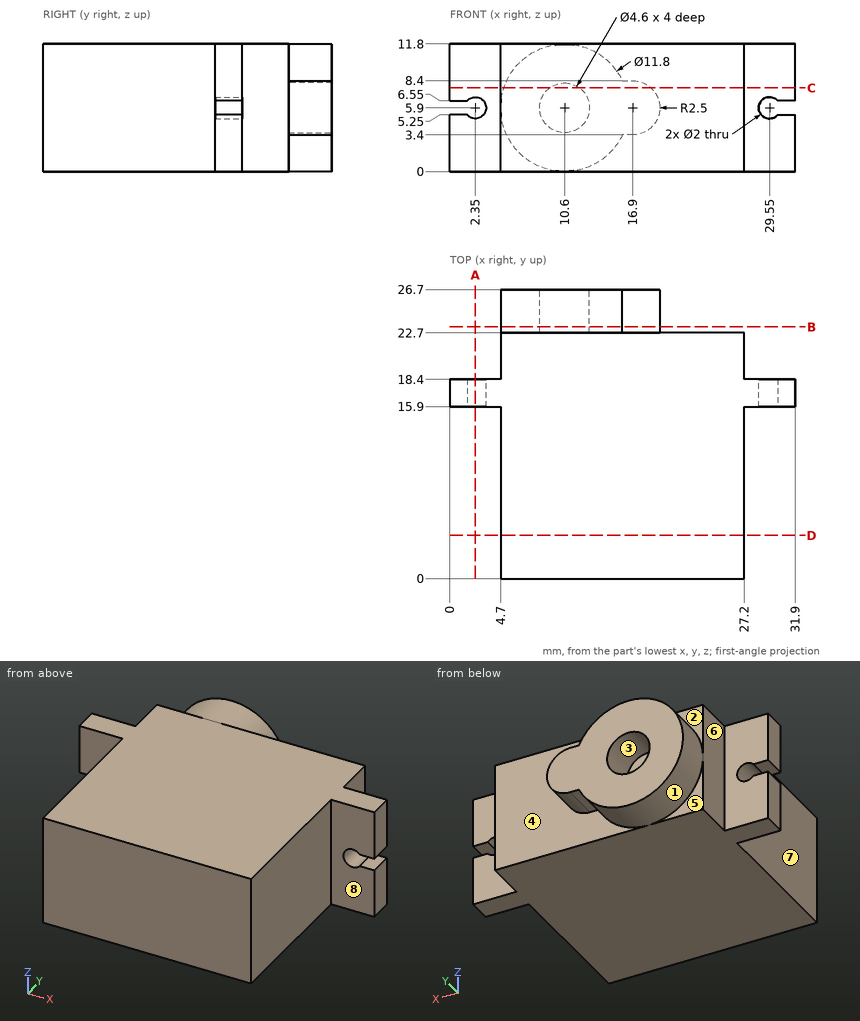
Design review of the part shown in the three views and the two pictorial views. Dimensions are in mm from the part's minimum x, y and z. A direction names the side the tool comes from. Round coordinates to 2 decimals unless told otherwise and drop trailing zeros. Write each loop counter-clockwise with the first axis right and the second up, starting at its lowest first coordinate (ties: lowest second). Pieces come first, ordered by that corner, then holes.
1) Take a section at C-C on z = 7.75. Give the boundary of the cut face in (x, y).
Answer below:
outline: (0, 15.9) - (4.7, 15.9) - (4.7, 0) - (27.2, 0) - (27.2, 15.9) - (31.9, 15.9) - (31.9, 18.4) - (27.2, 18.4) - (27.2, 22.7) - (18.58, 22.7) - (18.58, 26.7) - (11.97, 26.7) - (11.97, 22.7) - (9.23, 22.7) - (9.23, 26.7) - (5, 26.7) - (5, 22.7) - (4.7, 22.7) - (4.7, 18.4) - (0, 18.4) - close
2) Machinability: for the marked faces 4, 5, 6, 7 and 8, which of the approach directions +Z, -Z, +X, -X, +Y, -Y give a long, thin tool a straight path to every point of the face, cutting with its end or side? Answer none if there is none.
Answer below:
face 4: +X, +Y
face 5: -Z, -X, +Y
face 6: +Z, -Z, -X, +Y
face 7: +Z, -Z, -X, -Y
face 8: +Z, -Z, +X, -Y
3) Take a section at B-B on y = 23.25. Give the boundary of the cut face in (x, z), then the cut area to 3 significant figures.
Answer below:
outline: (15.94, 3.4) - (16.9, 3.4) arc R2.5 ccw to (16.9, 8.4) - (15.94, 8.4) arc R5.9 ccw (long way) to start; hole circle Ø4.6 at (10.6, 5.9)
area: 105 mm2
4) Mouldability with a two-part tool opening along Z and no side actions: class the marked faces 1, 2 and 3 as +Z half, -Z half, draft (parallel to the pull), parting line (faces both ways), or undercut.
Answer below:
face 1: parting line
face 2: draft
face 3: undercut
5) For line 1 along Z through (x, y) = (29.55, 16.8); line 2 along X through (y, z) = (24.55, 5.9); line 3 along Y through (x, z) = (26.5, 8), list the stretches that pass through material, from the lowest coordinate up.
Answer below:
line 1: z = 0 to 4.9, 6.9 to 11.8
line 2: x = 4.7 to 8.3, 12.9 to 19.4
line 3: y = 0 to 22.7
6) Insertion check: pin 1 Ø5 at (x, z) = (3, 8.5) entering from +Y; pin 2 Ø3.5 at (y, z) = (21.5, 8) entering from +X; pin 3 Ø1 at (y, z) = (21, 2) entering from -X; pin 4 Ø4 at (x, z) = (30.5, 8.5) entering from +Y. Each pin has a flat end and moves straight along its axis. Give the tip position at first contact, or say it passes through.
Answer below:
pin 1: stops at y = 26.7
pin 2: stops at x = 27.2
pin 3: stops at x = 4.7
pin 4: stops at y = 18.4
7) Take a section at D-D on y = 4. Give the boundary of the cut face in (x, z).
Answer below:
outline: (4.7, 0) - (27.2, 0) - (27.2, 11.8) - (4.7, 11.8) - close
8) Take a section at A-A on x = 2.35. Give the boundary of the cut face in (y, z), then the cut area to 3 significant figures.
Answer below:
outline: (15.9, 0) - (18.4, 0) - (18.4, 4.9) - (15.9, 4.9) - close; (15.9, 6.9) - (18.4, 6.9) - (18.4, 11.8) - (15.9, 11.8) - close
area: 24.5 mm2
